For this review, use the dimensioned drawing (mm, ordinates from the lowest corner) and the shaded views. A direction names the side the tool comes from. Coordinates: 2 decimals unless noted, no trailing zeros. Order: outer loops, then holes, each group sorted by start corner. A loop starts at its lowest first (then second) coordinate and runs counter-clockwise, first axis right, second up. Notation, with made-up numbers: M 5.5,75.25 L 14.5,75.25 A31 ccw 14.5,110.25 Z; hole C 23,37.5 d2. An arc over 180 degrees is marked long. Answer as CSV lines item,"result". Start each with the question number.
Q1. For P1, Ø1, axis at x = 47, z = 41, coming from the -Y side; P2, Ø7.5, axis at y = 19.5, z = 24.5, coming from the +X side; P3, Ø6, axis at x = 40, y = 41.5, coming from the +Z side; P4, Ø3, axis at x = 32.5, z = 24.5, coming from the -Y side, all flat-tipped, find the tip position at first contact; note any pin that passes through.
Q2. Machinability: for the marked faces 5, 6 and 7, which of the approach directions +Z, -Z, +X, -X, +Y, -Y give a long, thin tool a straight path to every point of the face, cutting with its end or side? Answer none if there is none.
Q3. Consider section C-C on x = 34.29. Write out the cut boundary in (y, z).
Q4. Consider section B-B on z = 43. Write out the cut boundary in (x, y).
Q5. Wall thickness on L1, parallel to X at y = 38, z = 40; L2, parallel to Y at x = 40.5, z = 18; L3, parallel to Z at x = 18, y = 25: over which ranges is each line inside the solid? List them lowest first. Write a range as [from, to].
Q6. Consider section D-D on y = 21.59. Write out the cut boundary in (x, z), and give its area (3 significant figures).
Q7. The part is to be moulded in two halves that separate along Y. For the marked faces 1, 2, 3 and 4, say which applies: +Y half, -Y half, draft (parallel to the pull), parting line (faces both ways), or undercut.
Q8. Consider section A-A on x = 19.5. Write out the cut boundary in (y, z) (1 decimal).
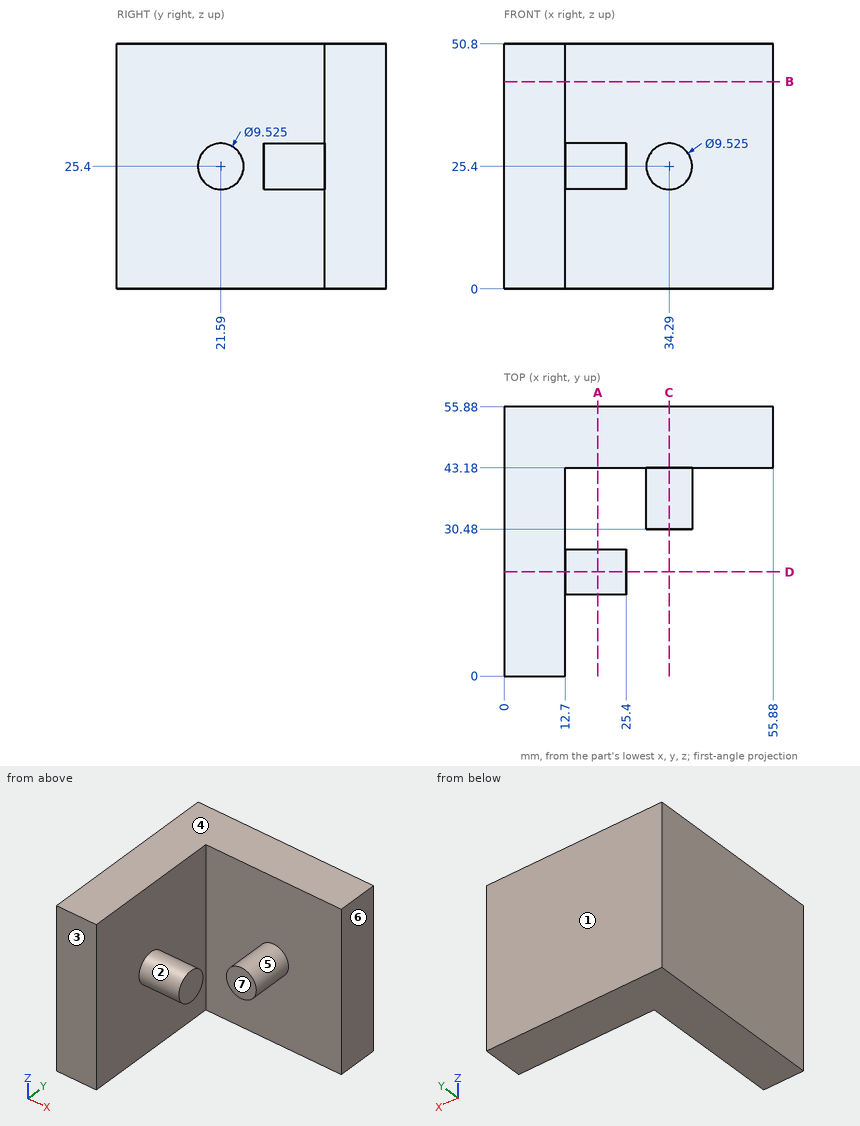
Evaluation:
1,P1,"stops at y = 43.18"
1,P2,"stops at x = 25.4"
1,P3,"stops at z = 50.8"
1,P4,"stops at y = 30.48"
2,face 5,"-Y"
2,face 6,"+Z, -Z, +X, +Y, -Y"
2,face 7,"+Z, -Z, +X, -Y"
3,outline,"M 30.48,20.64 L 43.18,20.64 L 43.18,0 L 55.88,0 L 55.88,50.8 L 43.18,50.8 L 43.18,30.16 L 30.48,30.16 Z"
4,outline,"M 0,0 L 12.7,0 L 12.7,43.18 L 55.88,43.18 L 55.88,55.88 L 0,55.88 Z"
5,L1,"x = [0, 12.7]"
5,L2,"y = [43.18, 55.88]"
5,L3,"z = [22.08, 28.72]"
6,outline,"M 0,0 L 12.7,0 L 12.7,20.64 L 25.4,20.64 L 25.4,30.16 L 12.7,30.16 L 12.7,50.8 L 0,50.8 Z"
6,area,"766 mm²"
7,face 1,"+Y half"
7,face 2,"undercut"
7,face 3,"-Y half"
7,face 4,"draft"
8,outline,"C 21.6,25.4 d9.5; M 43.2,0 L 55.9,0 L 55.9,50.8 L 43.2,50.8 Z"
